```python
from build123d import *

# Parameters (mm, degrees)
SALIENTE_EXTRUIR1_DEPTH = 6
CROQUIS2_W              = 21
CROQUIS2_H              = 41
CORTAR_EXTRUIR1_DEPTH   = 10
CROQUIS3_R              = 1
CORTAR_EXTRUIR2_DEPTH   = 10
CROQUIS4_R              = 2.25
CORTAR_EXTRUIR3_DEPTH   = 10
CROQUIS5_R              = 2.25
CORTAR_EXTRUIR4_DEPTH   = 10
CROQUIS9_R              = 2.25
CORTAR_EXTRUIR6_DEPTH   = 29
CROQUIS6_R              = 2.064168912
CROQUIS6_R_2            = 1.970714146
CROQUIS6_R_3            = 2.1
CORTAR_EXTRUIR7_DEPTH   = 10
REDONDEO1_R             = 6


with BuildPart() as part:
    # Croquis1 → Saliente-Extruir1 (new body)
    with BuildSketch(Plane(origin=(0, 0, 0), x_dir=(1, 0, 0), z_dir=(0, 1, 0))):
        Polygon((-55.627306273, -217.492892842), (-55.627306273, 12.564575646), (-5.627306273, 57.564575646), (-43.56277397, 85.075402887), (-43.56277397, 105.075421235), (-8.56277397, 132.507107158), (77.308161424, 132.507107158), (112.308161424, 105.074865922), (112.308161424, 85.073844823), (74.372693727, 57.564575646), (124.372693727, 12.564575646), (124.372693727, -217.492892842), align=None)
    extrude(amount=SALIENTE_EXTRUIR1_DEPTH)

    # Croquis2 → Cortar-Extruir1 (cut)
    with BuildSketch(Plane(origin=(0, 6, 0), x_dir=(1, 0, 0), z_dir=(0, 1, 0))):
        with Locations((34.372693727, 96.064575646)):
            Rectangle(CROQUIS2_W, CROQUIS2_H)
    extrude(amount=-CORTAR_EXTRUIR1_DEPTH, mode=Mode.SUBTRACT)

    # Croquis3 → Cortar-Extruir2 (cut)
    with BuildSketch(Plane(origin=(0, 6, 0), x_dir=(1, 0, 0), z_dir=(0, 1, 0))):
        with Locations((117.122693727, -177.492892842)):
            Circle(CROQUIS3_R)
        with Locations((117.122693727, -159.492892842)):
            Circle(CROQUIS3_R)
        with Locations((-48.377306273, -159.492892842)):
            Circle(CROQUIS3_R)
        with Locations((-48.377306273, -177.492892842)):
            Circle(CROQUIS3_R)
    extrude(amount=-CORTAR_EXTRUIR2_DEPTH, mode=Mode.SUBTRACT)

    # Croquis4 → Cortar-Extruir3 (cut)
    with BuildSketch(Plane(origin=(0, 6, 0), x_dir=(1, 0, 0), z_dir=(0, 1, 0))):
        with Locations((-16.877306273, -194.17563761)):
            Circle(CROQUIS4_R)
        with Locations((-16.877306273, -60.17563761)):
            Circle(CROQUIS4_R)
        with Locations((84.372693727, -60.17563761)):
            Circle(CROQUIS4_R)
        with Locations((84.372693727, -194.17563761)):
            Circle(CROQUIS4_R)
    extrude(amount=-CORTAR_EXTRUIR3_DEPTH, mode=Mode.SUBTRACT)

    # Croquis5 → Cortar-Extruir4 (cut)
    with BuildSketch(Plane(origin=(0, 6, 0), x_dir=(1, 0, 0), z_dir=(0, 1, 0))):
        with Locations((82.872693727, -51.34563761)):
            Circle(CROQUIS5_R)
        with Locations((-14.127306273, -51.34563761)):
            Circle(CROQUIS5_R)
        with Locations((-14.127306273, 41.07436239)):
            Circle(CROQUIS5_R)
        with Locations((82.872693727, 41.07436239)):
            Circle(CROQUIS5_R)
    extrude(amount=-CORTAR_EXTRUIR4_DEPTH, mode=Mode.SUBTRACT)

    # Croquis9 → Cortar-Extruir6 (cut)
    with BuildSketch(Plane(origin=(0, 0, 0), x_dir=(-1, 0, 0), z_dir=(0, -1, 0))):
        with Locations((-104.308161424, 94.983735042)):
            Circle(CROQUIS9_R)
        with Locations((35.56277397, 94.983735042)):
            Circle(CROQUIS9_R)
    extrude(amount=-CORTAR_EXTRUIR6_DEPTH, mode=Mode.SUBTRACT)

    # Croquis6 → Cortar-Extruir7 (cut)
    with BuildSketch(Plane(origin=(0, 0, 0), x_dir=(-1, 0, 0), z_dir=(0, -1, 0))):
        with Locations((-29.512693727, 120.689890176)):
            Circle(CROQUIS6_R)
        with Locations((-39.232693727, 120.725721264)):
            Circle(CROQUIS6_R_2)
        with Locations((-39.362693727, 71.26759894)):
            Circle(CROQUIS6_R_3)
        with Locations((-29.382693727, 71.26759894)):
            Circle(CROQUIS6_R_3)
    extrude(amount=-CORTAR_EXTRUIR7_DEPTH, mode=Mode.SUBTRACT)

    # Redondeo1
    redondeo1_edges = [part.edges().sort_by_distance(p)[0] for p in [
        (-55.627306273, 3, 217.492892842),
        (-55.627306273, 3, -12.564575646),
        (-5.627306273, 3, -57.564575646),
        (-43.56277397, 3, -85.075402887),
        (-43.56277397, 3, -105.075421235),
        (-8.56277397, 3, -132.507107158),
        (77.308161424, 3, -132.507107158),
        (112.308161424, 3, -105.074865922),
        (112.308161424, 3, -85.073844823),
        (74.372693727, 3, -57.564575646),
        (124.372693727, 3, -12.564575646),
        (124.372693727, 3, 217.492892842),
    ]]
    fillet(redondeo1_edges, radius=REDONDEO1_R)


solid = part.part
```
Geometry check sheet. Reference: the model listing, model coordinates, mm. A direction names the side the tool comes from. Round coordinates to 2 decimals unless told otherwise and drop trailing zeros. Use a Markdown table: item, result. Add a question column.
1) Set-up check for faces 4 (the flat face through (100.839, 2.958, -33.745)), 5 (the flat face through (-32.7, 3, -33.2)), 6 (the flat face through (34, 3, -75.565)), 7 (the flat face through (112.308, 3, -95)), 8 (the flat face through (36, 6, 40)): record each of +Z, -Z, +X, -X, +Y, -Y from which the full face is reachable in a straight line by a thin tool's end or side.
2) Gauge pin test, flat ends, axial feed: P1, Ø1.5, axis at y = 0.5, z = -37, coming from the -X side; P2, Ø3, axis at y = 4, z = -96, coming from the +X side; P3, Ø1.5, axis at y = 1.5, z = -47, coming from the +X side. Record the tip position at first contact, or that the pin passes through.
3) Mould release check, pull along Z, two halves, no side actions. Record for faces 1 (the flat face through (-43.563, 3, -95)), 2 (the flat face through (44.873, 3, -96)), 3 (the cylindrical face through (-53.916, 3.042, 215.689)): released by +Z, released by -Z, zero draft, split by the parting line, or undercut.
4) Thickness scan on line 1 along Z through (x, y) = (117, 3.3); line 2 along Z through (x, y) = (-18.5, 2.4); line 3 along X through (y, z) = (4.4, 160). Record the ranges inside material, lowest first.
5) Section check A-A (y = 3.45). Count the separate pieces of the cut face and the enclosed holes in it, then the cut area to 3 significant figures.
Established:
| question | item | result |
|---|---|---|
| 1 | face 4 | +X, +Y, -Y |
| 1 | face 5 | -X, +Y, -Y |
| 1 | face 6 | +Y, -Y |
| 1 | face 7 | -Z, +X, +Y, -Y |
| 1 | face 8 | +Z, -Z, +X, -X, +Y |
| 2 | P1 | x = -29.31 |
| 2 | P2 | x = 112.31 |
| 2 | P3 | x = 86.94 |
| 3 | face 1 | zero draft |
| 3 | face 2 | undercut |
| 3 | face 3 | released by +Z |
| 4 | line 1 | -19.2 to 158.5, 160.49 to 176.5, 178.49 to 217.49 |
| 4 | line 2 | -124.72 to -66.9, -45.98 to 58.62, 61.73 to 192.62, 195.73 to 217.49 |
| 4 | line 3 | -55.63 to -49.24, -47.52 to 116.26, 117.98 to 124.37 |
| 5 | separate pieces | 1 |
| 5 | enclosed holes | 19 |
| 5 | area | 55,900 mm2 |
